```python
from build123d import *

# Parameters (mm, degrees)
SKETCH1_W           = 30
SKETCH1_H           = 30
BOSS_EXTRUDE1_DEPTH = 14
SKETCH2_R           = 1.7
CUT_EXTRUDE1_DEPTH  = 12
CUT_EXTRUDE2_DEPTH  = 11
FILLET1_R           = 0.7
FILLET2_R           = 0.5
FILLET3_R           = 0.8
FILLET4_R           = 0.8


# Some blends are built 0.0001 mm under size
with BuildPart() as part:
    # Sketch1 → Boss-Extrude1 (new body)
    with BuildSketch(Plane(origin=(0, 0, 0), x_dir=(1, 0, 0), z_dir=(0, 1, 0))):
        Rectangle(SKETCH1_W, SKETCH1_H)
    extrude(amount=BOSS_EXTRUDE1_DEPTH)

    # Sketch2 → Cut-Extrude1 (cut)
    with BuildSketch(Plane(origin=(0, 14, 0), x_dir=(1, 0, 0), z_dir=(0, 1, 0))):
        with Locations(Location((0, 0, 0), (0, 0, 270))):
            Circle(SKETCH2_R)
    extrude(amount=-CUT_EXTRUDE1_DEPTH, mode=Mode.SUBTRACT)

    # Sketch3 → Cut-Extrude2 (cut)
    with BuildSketch(Plane(origin=(0, 14, 0), x_dir=(1, 0, 0), z_dir=(0, 1, 0))):
        Polygon((2.095936352, 2.803043133), (12.792893219, 13.5), (0.5, 13.5), (0.5, 3.464101615), align=None)
        Polygon((2.803043133, 2.095936352), (13.5, 12.792893219), (13.5, 0.5), (3.464101615, 0.5), align=None)
        Polygon((3.464101615, -0.5), (13.5, -0.5), (13.5, -12.792893219), (2.803043133, -2.095936352), align=None)
        Polygon((2.095936352, -2.803043133), (12.792893219, -13.5), (0.5, -13.5), (0.5, -3.464101615), align=None)
        Polygon((-2.095936352, -2.803043133), (-12.792893219, -13.5), (-0.5, -13.5), (-0.5, -3.464101615), align=None)
        Polygon((-2.803043133, -2.095936352), (-13.5, -12.792893219), (-13.5, -0.5), (-3.464101615, -0.5), align=None)
        Polygon((-2.803043133, 2.095936352), (-13.5, 12.792893219), (-13.5, 0.5), (-3.464101615, 0.5), align=None)
        Polygon((-2.095936352, 2.803043133), (-12.792893219, 13.5), (-0.5, 13.5), (-0.5, 3.464101615), align=None)
    extrude(amount=-CUT_EXTRUDE2_DEPTH, mode=Mode.SUBTRACT)

    # Fillet1
    fillet1_edges = [part.edges().sort_by_distance(p)[0] for p in [
        (0, 14, -1.7),
    ]]
    fillet(fillet1_edges, radius=FILLET1_R)

    # Fillet2
    fillet2_edges = [part.edges().sort_by_distance(p)[0] for p in [
        (0, 14, 15),
        (15, 14, 0),
        (8.482050808, 14, -0.5),
        (13.5, 14, -6.646446609),
        (8.151521567, 14, -7.444414786),
        (3.133572374, 14, -1.297968176),
        (-0.5, 14, 8.482050808),
        (-1.297968176, 14, 3.133572374),
        (-7.444414785, 14, 8.151521567),
        (-6.646446609, 14, 13.5),
        (0.5, 14, -8.482050808),
        (1.297968176, 14, -3.133572374),
        (7.444414786, 14, -8.151521567),
        (6.646446609, 14, -13.5),
        (0, 14, -15),
        (0.5, 14, 8.482050808),
        (6.646446609, 14, 13.5),
        (7.444414786, 14, 8.151521567),
        (1.297968176, 14, 3.133572374),
        (-8.482050808, 14, 0.5),
        (-13.5, 14, 6.646446609),
        (-8.151521567, 14, 7.444414786),
        (-3.133572374, 14, 1.297968176),
        (-8.482050808, 14, -0.5),
        (-3.133572374, 14, -1.297968176),
        (-8.151521567, 14, -7.444414786),
        (-13.5, 14, -6.646446609),
        (13.5, 14, 6.646446609),
        (8.482050808, 14, 0.5),
        (3.133572374, 14, 1.297968176),
        (8.151521567, 14, 7.444414786),
        (-0.5, 14, -8.482050808),
        (-6.646446609, 14, -13.5),
        (-7.444414786, 14, -8.151521567),
        (-1.297968176, 14, -3.133572374),
        (-15, 14, 0),
    ]]
    fillet(fillet2_edges, radius=FILLET2_R - 0.0001)  # a hair under: the kernel refuses the full size

    # Fillet3
    fillet3_edges = [part.edges().sort_by_distance(p)[0] for p in [
        (15, 0, 0),
        (0, 0, 15),
        (-15, 0, 0),
        (0, 0, -15),
    ]]
    fillet(fillet3_edges, radius=FILLET3_R)

    # Fillet4
    # the kernel refuses this fillet: 0.8 mm, written as the material it takes off along each edge
    with BuildSketch(Plane(origin=(-14.2, 14, 14.2), x_dir=(-1, 0, 0), z_dir=(0, 0, -1))) as fillet4_piece_1:
        with BuildLine():
            CenterArc((0.3001, -0.4999), 0.4999, 0, 90)
            Line((0.8, -0.4999), (0.8, 0))
            Line((0.8, 0), (0.3001, 0))
        make_face()
    revolve(axis=Axis((-14.2, 14, 14.2), (0, 1, 0)), revolution_arc=90, mode=Mode.SUBTRACT)
    with BuildSketch(Plane(origin=(-14.2, 14, -14.2), x_dir=(0, 0, -1), z_dir=(1, 0, 0))) as fillet4_piece_2:
        with BuildLine():
            CenterArc((0.3001, -0.4999), 0.4999, 0, 90)
            Line((0.8, -0.4999), (0.8, 0))
            Line((0.8, 0), (0.3001, 0))
        make_face()
    revolve(axis=Axis((-14.2, 14, -14.2), (0, 1, 0)), revolution_arc=90, mode=Mode.SUBTRACT)
    with BuildSketch(Plane(origin=(14.2, 14, 14.2), x_dir=(0, 0, 1), z_dir=(-1, 0, 0))) as fillet4_piece_3:
        with BuildLine():
            CenterArc((0.3001, -0.4999), 0.4999, 0, 90)
            Line((0.8, -0.4999), (0.8, 0))
            Line((0.8, 0), (0.3001, 0))
        make_face()
    revolve(axis=Axis((14.2, 14, 14.2), (0, 1, 0)), revolution_arc=90, mode=Mode.SUBTRACT)
    with BuildSketch(Plane(origin=(14.2, 14, -14.2), x_dir=(1, 0, 0), z_dir=(0, 0, 1))) as fillet4_piece_4:
        with BuildLine():
            CenterArc((0.3001, -0.4999), 0.4999, 0, 90)
            Line((0.8, -0.4999), (0.8, 0))
            Line((0.8, 0), (0.3001, 0))
        make_face()
    revolve(axis=Axis((14.2, 14, -14.2), (0, 1, 0)), revolution_arc=90, mode=Mode.SUBTRACT)
    with BuildSketch(Plane(origin=(14.2, 0.8, 14.2), x_dir=(1, 0, 0), z_dir=(0, 0, 1))) as fillet4_piece_5_section:
        Polygon((0, 0), (FILLET4_R, 0), (FILLET4_R, -FILLET4_R), (0, -FILLET4_R), align=None)
    fillet4_piece_5 = extrude(amount=FILLET4_R, mode=Mode.PRIVATE)
    fillet4_piece_5 = fillet4_piece_5 - Plane(origin=(14.2, 0.8, 14.2), x_dir=(-0.7071067811865475, 0.7071067811865475, 0), z_dir=(0, 0, 1)) * Sphere(FILLET4_R, mode=Mode.PRIVATE)
    add(fillet4_piece_5, mode=Mode.SUBTRACT)
    with BuildSketch(Plane(origin=(14.2, 0.8, -14.2), x_dir=(0, 0, -1), z_dir=(1, 0, 0))) as fillet4_piece_6_section:
        Polygon((0, 0), (FILLET4_R, 0), (FILLET4_R, -FILLET4_R), (0, -FILLET4_R), align=None)
    fillet4_piece_6 = extrude(amount=FILLET4_R, mode=Mode.PRIVATE)
    fillet4_piece_6 = fillet4_piece_6 - Plane(origin=(14.2, 0.8, -14.2), x_dir=(0, 0.7071067811865475, 0.7071067811865475), z_dir=(1, 0, 0)) * Sphere(FILLET4_R, mode=Mode.PRIVATE)
    add(fillet4_piece_6, mode=Mode.SUBTRACT)
    with BuildSketch(Plane(origin=(-14.2, 0.8, 14.2), x_dir=(-1, 0, 0), z_dir=(0, 0, 1))) as fillet4_piece_7_section:
        Polygon((0, 0), (FILLET4_R, 0), (FILLET4_R, FILLET4_R), (0, FILLET4_R), align=None)
    fillet4_piece_7 = extrude(amount=FILLET4_R, mode=Mode.PRIVATE)
    fillet4_piece_7 = fillet4_piece_7 - Plane(origin=(-14.2, 0.8, 14.2), x_dir=(0.7071067811865475, 0.7071067811865475, 0), z_dir=(0, 0, 1)) * Sphere(FILLET4_R, mode=Mode.PRIVATE)
    add(fillet4_piece_7, mode=Mode.SUBTRACT)
    with BuildSketch(Plane(origin=(-14.2, 0.8, -14.2), x_dir=(0, 0, -1), z_dir=(-1, 0, 0))) as fillet4_piece_8_section:
        Polygon((0, 0), (FILLET4_R, 0), (FILLET4_R, FILLET4_R), (0, FILLET4_R), align=None)
    fillet4_piece_8 = extrude(amount=FILLET4_R, mode=Mode.PRIVATE)
    fillet4_piece_8 = fillet4_piece_8 - Plane(origin=(-14.2, 0.8, -14.2), x_dir=(0, 0.7071067811865475, 0.7071067811865475), z_dir=(-1, 0, 0)) * Sphere(FILLET4_R, mode=Mode.PRIVATE)
    add(fillet4_piece_8, mode=Mode.SUBTRACT)
    with BuildSketch(Plane(origin=(15, 0.8, -15), x_dir=(0, 0, 1), z_dir=(0, 1, 0)), Plane(origin=(15, 0.8, 15), x_dir=(-1, 0, 0), z_dir=(0, 1, 0))) as fillet4_piece_9:
        with BuildLine():
            CenterArc((FILLET4_R, -FILLET4_R), FILLET4_R, 90, 90)
            Line((0, -FILLET4_R), (0, 0))
            Line((0, 0), (FILLET4_R, 0))
        make_face()
    extrude(amount=13.2, mode=Mode.SUBTRACT)
    with BuildSketch(Plane(origin=(-15, 0.8, 15), x_dir=(1, 0, 0), z_dir=(0, 1, 0)), Plane(origin=(-15, 0.8, -15), x_dir=(0, 0, 1), z_dir=(0, 1, 0))) as fillet4_piece_10:
        with BuildLine():
            CenterArc((FILLET4_R, FILLET4_R), FILLET4_R, 180, 90)
            Line((0, FILLET4_R), (0, 0))
            Line((0, 0), (FILLET4_R, 0))
        make_face()
    extrude(amount=13.2, mode=Mode.SUBTRACT)


solid = part.part
```
Build history of the part. All positions in model axes, mm. A direction names the side the tool comes from. Give positions to 0.01 mm unless a question says otherwise; leave off trailing zeros. Write item = value, one per line. Start each with the question number.
(1) Two-plate mould, pull along X, no slides. Class faces 3 (the cylindrical face through (-7.942, 13.857, -8.436)), 4 (the flat face through (0, 0, 0)), 5 (the cylindrical face through (-14.77, 0.24, -0.2)), 6 (the flat face through (7, 8, 13.5)): released by +X, released by -X, zero draft, split by the parting line, or undercut.
(2) Which spindle directions (+Z, -Z, +X, -X, +Y, -Y) get a long thin tool onto all of the face, cutting with end or side? Do faces 1 (the cylindrical face through (14.76, 7.06, 14.77)), 2 (the cylindrical face through (7.942, 13.857, -8.436)). Say none if no direction does.
(3) Pin check, flat tips, straight feed: pin 1 Ø1 at (x, z) = (0.5, -0.5) entering from +Y; pin 2 Ø3 at (x, z) = (9, -5) entering from +Y; pin 3 Ø8.5 at (x, z) = (-6, 8.5) entering from +Y. Stop position of each tip, or through.
(4) Probe L1, parallel to Z at x = 8, y = 13.25; L2, parallel to Z at x = 4.5, y = 5; L3, parallel to X at y = 10.5, z = 7.25. List the from-to ranges inside material, lowest first. Write a range as [from, to].
(5) Slice it at A-A on y = 7.75. State how many separate pieces and enclosed holes the cut face has, plus the area to 3 significant figures.
Responses:
q1.face_3 = undercut
q1.face_4 = zero draft
q1.face_5 = released by -X
q1.face_6 = undercut
q2.face_1 = +Z, +X, +Y, -Y
q2.face_2 = +Y
q3.pin_1 = 2
q3.pin_2 = 3
q3.pin_3 = 14
q4.L1 = [-15, -13.5], [-8.71, -7.29], [-0.5, 0.5], [7.29, 8.71], [13.5, 15]
q4.L2 = [-15, -13.5], [-5.21, -3.79], [-0.5, 0.5], [3.79, 5.21], [13.5, 15]
q4.L3 = [-15, -13.5], [-7.96, -6.54], [-0.5, 0.5], [6.54, 7.96], [13.5, 15]
q5.separate_pieces = 1
q5.enclosed_holes = 9
q5.area = 300 mm2
